Autodesk Inventor part; units mm, degrees
ref_plane "YZ Plane" through (0, 0, 0) normal (1, 0, 0) x (0, 1, 0)
ref_plane "XZ Plane" through (0, 0, 0) normal (0, 1, 0) x (-1, 0, 0)
ref_plane "XY Plane" through (0, 0, 0) normal (0, 0, 1) x (1, 0, 0)
sketch "Sketch1" plane through (0, 0, 0) normal (0, 1, 0) x (-1, 0, 0)
  circle A0 centre (0, 0) radius 89 construction
  circle A1 centre (0, 0) radius 104 construction
  circle A2 centre (0, 0) radius 157.5 construction
  circle A3 centre (0, 0) radius 172.5 construction
  circle A4 centre (0, 0) radius 96.5 construction
  circle A5 centre (0, 0) radius 165 construction
  line L0 (0, 0) -> (0, -209.0924)
  line L1 (0, 0) -> (71.5138, -196.4826)
  line L2 (0, 0) -> (134.402, -160.1741)
  line L3 (0, 0) -> (181.0793, -104.5462)
  line L4 (0, 0) -> (205.9158, -36.3085)
  line L5 (0, 0) -> (205.9158, 36.3085)
  line L6 (0, 0) -> (181.0793, 104.5462)
  line L7 (0, 0) -> (134.402, 160.1741)
  line L8 (0, 0) -> (71.5138, 196.4826)
  line L9 (0, 0) -> (0, 209.0924)
  line L10 (0, 0) -> (-71.5138, 196.4826)
  line L11 (0, 0) -> (-134.402, 160.1741)
  line L12 (0, 0) -> (-181.0793, 104.5462)
  line L13 (0, 0) -> (-205.9158, 36.3085)
  line L14 (0, 0) -> (-205.9158, -36.3085)
  line L15 (0, 0) -> (-181.0793, -104.5462)
  line L16 (0, 0) -> (-134.402, -160.1741)
  line L17 (0, 0) -> (-71.5138, -196.4826)
  circle A6 centre (33.0049, -90.6803) radius 1.75
  circle A7 centre (56.4333, -155.0493) radius 1.75
  circle A8 centre (0, -96.5) radius 1.75
  circle A9 centre (0, -165) radius 1.75
  line L18 (0, 0) -> (86.25, -149.3894)
  line L19 (0, 0) -> (-29.9543, -169.8793)
  arc A10 (-29.9543, -169.8793) -> (86.25, -149.3894) centre (0, 0) ccw
  arc A11 (-15.4547, -87.6479) -> (44.5, -77.0763) centre (0, 0) ccw
  arc A12 (-18.0594, -102.42) -> (52, -90.0666) centre (0, 0) ccw
  arc A13 (-27.3496, -155.1072) -> (78.75, -136.399) centre (0, 0) ccw
  line L20 (0, 0) -> (25.4898, -144.5597)
  arc A14 (-8.5012, -129.7217) -> (33.7594, -125.5401) centre (0, 0) ccw
  circle A15 centre (22.5743, -128.025) radius 1.75
  dimension "d0" = 178
  dimension "d1" = 208
  dimension "d2" = 315
  dimension "d3" = 345
  dimension "d4" = 193
  dimension "d5" = 330
  dimension "d8" = 360
  dimension "d11" = 3.5
  dimension "d13" = 3.5
  dimension "d14" = 3.5
  dimension "d15" = 3.5
  dimension "d23" = 10
  dimension "d24" = 10
  dimension "d25" = 20
  dimension "d26" = 130
  dimension "d27" = 3.5
extrude "Extrusion1" add sketch "Sketch1" along normal blind 5 contours A11 L20 A12 L0 A8 | L0 A8 A12 L19 A11 | A11 L18 A12 L1 A6 | L1 A6 A12 L20 A11 | L18 A10 L1 A7 A13 | A13 L0 A9 A10 L19 | L1 A7 A10 L0 A9 A13
extrude "Extrusion2" add sketch "Sketch1" along normal blind 2 contours L18 A13 L1 A12 | A12 L0 A13 L19 | L20 A15 A14 L0 A12 | A12 L1 A13 L0 A14 A15 L20 | A15 A14 L20 | L20 A14 A15 | A14 A15 L20 | L20 A15 A14
chamfer "Chamfer1" distance 2 angle 45 4 edges at (1.75, 0, -96.5) (1.75, 0, -165) (-54.6833, 0, -155.0493) (-31.2549, 0, -90.6803)
extrude "Extrusion3" cut sketch "Sketch1" along normal through all contours A15 A14 L20 | L20 A14 A15 | A14 A15 L20 | L20 A15 A14
chamfer "Chamfer2" distance 2 angle 45 1 edges at (-20.8243, 2, -128.025)
properties part number "stator-bottom-connector"
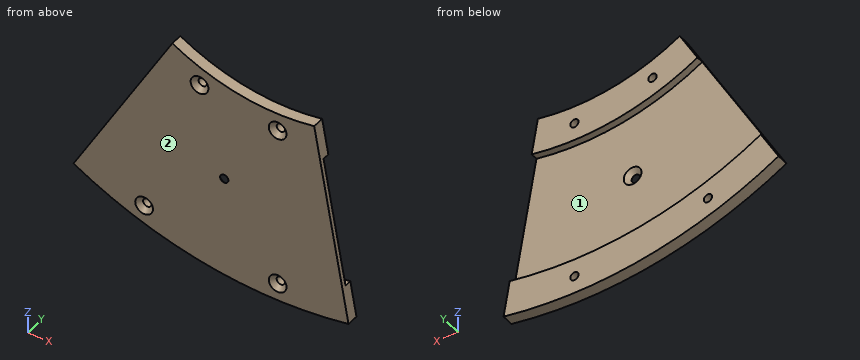
The model under review builds one solid part; all positions refer to its coordinate system, in mm. Face numbers are marked on the shaded views. Coordinates: 2 decimals unless noted, no trailing zeros. Loops run counter-clockwise (first coordinate to the right, second up) from the corner with the lowest first, then second, coordinate; pieces in that order, holes last. Notation, with made-up numbers: M 44.5,17 L 66.5,17 A11 ccw 66.5,33 Z; hole C 84,-31 d1. An arc over 180 degrees is marked long. Put each result on its own line as item: value. Start each with the question number.
Q1. Add section B-B (z = -165). Write out the cut boundary in (x, y).
Q2. Clearance check with flat-ended pins moving along their axes: pin 1 (8 mm diameter, centred on x = -5, z = -151, fed in from +Y); pin 2 (3 mm diameter, centred on x = -9, y = 1.5, fed in from +Z); pin 3 (4 mm diameter, centred on x = -33, z = -90.68, fed in from -Y). State where each tip first meets the part, or that it passes through.
Q3. Add section A-A (x = 0). Write out the cut boundary in (y, z).
Q4. Wall thickness on line 1 (Z direction, x = 0, y = 4.2); line 2 (Z direction, x = 1.5, y = 4.85); line 3 (Y direction, x = -4.5, z = -144): over which ranges is each line inside the solid? List them lowest first.
Q5. Add section C-C (y = 2.9). Write out the cut boundary in (x, z), and give its area (3 significant figures).
Q6. Add section D-D (x = -14.5). Write out the cut boundary in (y, z).
Q7. The part is to be moulded in two halves that separate along Z. For the marked faces 1 and 2, say which applies: +Z half, -Z half, draft (parallel to the pull), parting line (faces both ways), or undercut.
Answers:
1. outline: M -50.31,0 L -3.75,0 L -1.75,2 L -1.75,5 L -50.31,5 Z; M 1.75,2 L 3.75,0 L 29.09,0 L 29.09,5 L 1.75,5 Z
2. pin 1: stops at y = 2
2. pin 2: stops at z = -88.38
2. pin 3: stops at y = 1.75
3. outline: M 0,-172.5 L 5,-172.5 L 5,-166.75 L 2,-166.75 L 0,-168.75 Z; M 0,-161.25 L 2,-163.25 L 5,-163.25 L 5,-157.5 L 2,-157.5 L 2,-104 L 5,-104 L 5,-98.25 L 2,-98.25 L 0,-100.25 Z; M 0,-92.75 L 2,-94.75 L 5,-94.75 L 5,-89 L 0,-89 Z
4. line 1: z = -172.5 to -166.75, -163.25 to -157.5, -104 to -98.25, -94.75 to -89
4. line 2: z = -172.49 to -165.9, -164.1 to -157.49, -103.99 to -97.4, -95.6 to -88.99
4. line 3: y = 0 to 2
5. outline: M -86.25,-149.39 A172.5 ccw 29.95,-169.88 L 27.35,-155.11 A157.5 cw -78.75,-136.4 Z; M -52,-90.07 A104 ccw 18.06,-102.42 L 15.45,-87.65 A89 cw -44.5,-77.08 Z; hole C -56.43,-155.05 d3.5; hole C -33,-90.68 d3.5; hole C 0,-165 d3.5; hole C 0,-96.5 d3.5
5. area: 2,700 mm^2
6. outline: M 0,-171.89 L 5,-171.89 L 5,-156.83 L 2,-156.83 L 2,-102.98 L 5,-102.98 L 5,-87.81 L 0,-87.81 Z
7. face 1: undercut
7. face 2: draft
